Check sheet for the modelled part. Datum: model origin and axes. Units: mm. A direction names the side the tool comes from. Give positions to 0.01 mm unless a question says otherwise; leave off trailing zeros. Order: outer loops, then holes, each group sorted by start corner. A loop starts at its lowest first (then second) coordinate and runs counter-clockwise, first axis right, second up. Notation, with made-up numbers: M 8,-24.75 L 21,-24.75 A29 ccw 21,-3.75 Z; hole C 79.25,-30 d4. An arc over 180 degrees is marked long. Answer in a Markdown table with one row per item. Add a question column.
from build123d import *

# Parameters (mm, degrees)
F3_DEPTH = 36.5125
F5_D     = 7.9375
F5_DEPTH = 36.5125
F5_TIP   = 2.3846655818


with BuildPart() as f1:
    # F0 (on Front) → F1 (revolve)
    with BuildSketch(Plane.XZ):
        Polygon((-342.9, 38.1), (-342.9, 0), (342.9, 0), (342.9, 19.05), (-292.1, 19.05), (-292.1, 38.1), align=None)
    revolve(axis=Axis((0, 0, 0), (-1, 0, 0)))

    # F2 (on face) → F3 (join)
    with BuildSketch(Plane.YZ.offset(342.9)):
        Polygon((5.499261314, 9.525), (-5.499261314, 9.525), (-10.9985226281, 0), (-5.499261314, -9.525), (5.499261314, -9.525), (10.9985226281, 0), align=None)
    extrude(amount=F3_DEPTH)

    # F5
    with Locations(Plane.YZ.offset(379.4125)):
        with Locations((0, 0)):
            Hole(F5_D / 2, depth=F5_DEPTH)
            with Locations((0, 0, -(F5_DEPTH + F5_TIP / 2))):  # 118° drill point
                Cone(0, F5_D / 2, F5_TIP, mode=Mode.SUBTRACT)


solid = f1.part
Q1. Tool access check on faces 1 (the flat face through (361, 0, 9.525)), 2 (the flat face through (361, 0, -9.525)), 3 (the flat face through (-292.1, 17.5, -7.9)). Record the directions out of +Z, -Z, +X, -X, +Y, -Y that give a thin tool (end or side, any length) a straight path to the whole face; none if there is none.
Q2. Cross-section at C-C (x = 101). Record the boundary of the cut face in (y, z), and give its area (3 significant figures).
Q3. Go/stop test with flat-tipped pins: pin 1 (1.5 mm diameter, centred on y = -18.5, z = 8.5, fed in from +X); pin 2 (6 mm diameter, centred on x = 226.5, y = -1.5, fed in from +Z); pin 3 (5.5 mm diameter, centred on x = 355.5, y = 2, fed in from -Z) (3 decimals); pin 4 (12.5 mm diameter, centred on y = 0, z = 0, fed in from +X). Record where each tip stops, or that it passes through.
Q4. Cross-section at B-B (y = 31.5). Record the boundary of the cut face in (x, z), and give its area (3 significant figures).
Q5. Cross-section at A-A (z = 28). Record the boundary of the cut face in (x, y).
Q6. Thickness scan on probe 1 along Y at (x, z) = (363.5, 0); probe 2 along Z at (x, y) = (365, 0) (3 decimals); probe 3 along X at (y, z) = (25, -8). Record the ranges inside material, lowest first.
Values follow:
| question | item | result |
|---|---|---|
| 1 | face 1 | +Z, +X, +Y, -Y |
| 1 | face 2 | -Z, +X, +Y, -Y |
| 1 | face 3 | +X |
| 2 | outline | C 0,0 d38.1 |
| 2 | area | 1,140 mm² |
| 3 | pin 1 | x = -292.1 |
| 3 | pin 2 | z = 19.05 |
| 3 | pin 3 | z = -9.525 |
| 3 | pin 4 | x = 379.41 |
| 4 | outline | M -342.9,-21.43 L -292.1,-21.43 L -292.1,21.43 L -342.9,21.43 Z |
| 4 | area | 2,180 mm² |
| 5 | outline | M -342.9,-25.84 L -292.1,-25.84 L -292.1,25.84 L -342.9,25.84 Z |
| 6 | probe 1 | -11 to -3.97, 3.97 to 11 |
| 6 | probe 2 | -9.525 to -3.969, 3.969 to 9.525 |
| 6 | probe 3 | -342.9 to -292.1 |
